Can you work these out from the model? Positions are in its coordinate system, mm. A direction names the side the tool comes from. Give positions to 0.01 mm unless a question says otherwise; leave off trailing zeros. Loops run counter-clockwise (first coordinate to the right, second up) from the corner with the lowest first, then second, coordinate; pieces in that order, holes last. Notation, with made-up numbers: M 85.5,43 L 119.5,43 A32 cw 119.5,82 Z; hole C -10.5,46 d1. An arc over 180 degrees is marked long. Put each result on its own line as item: value. Start each with the question number.
1) Imagine slicing it at D-D (y = -100). Write out the boundary of the cut face in (x, z), then the cut area to 3 significant figures.
2) Imagine slicing it at B-B (z = 51). Write out the boundary of the cut face in (x, y).
3) Please list where these lines run through material, in increasing order: line 1 along X through (y, z) = (46, 70); line 2 along Z through (x, y) = (-191, -99); line 3 along Y through (x, z) = (109, 81.5). Write a range as from..to.
4) For faces 1 (the cylindrical face through (-156.99, -82.15, 65.42)), 2 (the flat face through (-2, 85, 65)), 3 (the flat face through (-160, -1, 65)), which set-ups out of +Z, -Z, +X, -X, +Y, -Y let a thin tool reach every point of the face, with its end or its side?
5) Imagine slicing it at A-A (x = 40.5). Write out the boundary of the cut face in (y, z).
6) For P1, Ø1.5, axis at x = -157, y = -80, coming from the +Z side; P2, Ø2, axis at x = -93, y = 85, coming from the +Z side; P3, Ø18, axis at x = -11, z = 66, coming from the -Y side, each with a flat end and sliding along its axis, tell me the tip position at first contact or that it passes through.
7) Imagine slicing it at C-C (y = -29.5). Write out the boundary of the cut face in (x, z).
from build123d import *

# Parameters (mm, degrees)
F0_W     = 500
F0_H     = 250
F1_DEPTH = 25
F2_W     = 320
F2_H     = 170
F3_DEPTH = 80
F4_R     = 10
F5_SIZE  = 10


with BuildPart() as f1:
    # F0 (on Top) → F1 (new body, symmetric)
    with BuildSketch(Plane.XY):
        Rectangle(F0_W, F0_H)
    extrude(amount=F1_DEPTH, both=True)

    # F2 (on face) → F3 (join)
    with BuildSketch(Plane.XY.offset(25)):
        Rectangle(F2_W, F2_H)
    extrude(amount=F3_DEPTH)

    # F4
    f4_edges = [f1.edges().sort_by_distance(p)[0] for p in [
        (0, -85, 105),
        (160, 0, 105),
        (0, 85, 105),
        (-160, 0, 105),
        (-160, -85, 65),
        (160, -85, 65),
        (160, 85, 65),
        (-160, 85, 65),
        (-160, 0, 25),
        (0, -85, 25),
        (160, 0, 25),
        (0, 85, 25),
    ]]
    fillet(f4_edges, radius=F4_R)

    # F5
    f5_edges = [f1.edges().sort_by_distance(p)[0] for p in [
        (-250, -125, 0),
        (-250, 125, 0),
        (250, 125, 0),
        (250, -125, 0),
    ]]
    chamfer(f5_edges, length=F5_SIZE)


solid = f1.part
Recorded:
1. outline: M -250,-25 L 250,-25 L 250,25 L -250,25 Z
1. area: 25,000 mm²
2. outline: M -160,-75 A10 ccw -150,-85 L 150,-85 A10 ccw 160,-75 L 160,75 A10 ccw 150,85 L -150,85 A10 ccw -160,75 Z
3. line 1: -160..160
3. line 2: -25..25
3. line 3: -85..85
4. face 1: +Z, -X, -Y
4. face 2: +Z, +X, -X, +Y
4. face 3: +Z, -X, +Y, -Y
5. outline: M -125,-25 L 125,-25 L 125,25 L 95,25 A10 cw 85,35 L 85,95 A10 ccw 75,105 L -75,105 A10 ccw -85,95 L -85,35 A10 cw -95,25 L -125,25 Z
6. P1: z = 101.19
6. P2: z = 99.36
6. P3: y = -85
7. outline: M -250,-25 L 250,-25 L 250,25 L 170,25 A10 cw 160,35 L 160,95 A10 ccw 150,105 L -150,105 A10 ccw -160,95 L -160,35 A10 cw -170,25 L -250,25 Z
